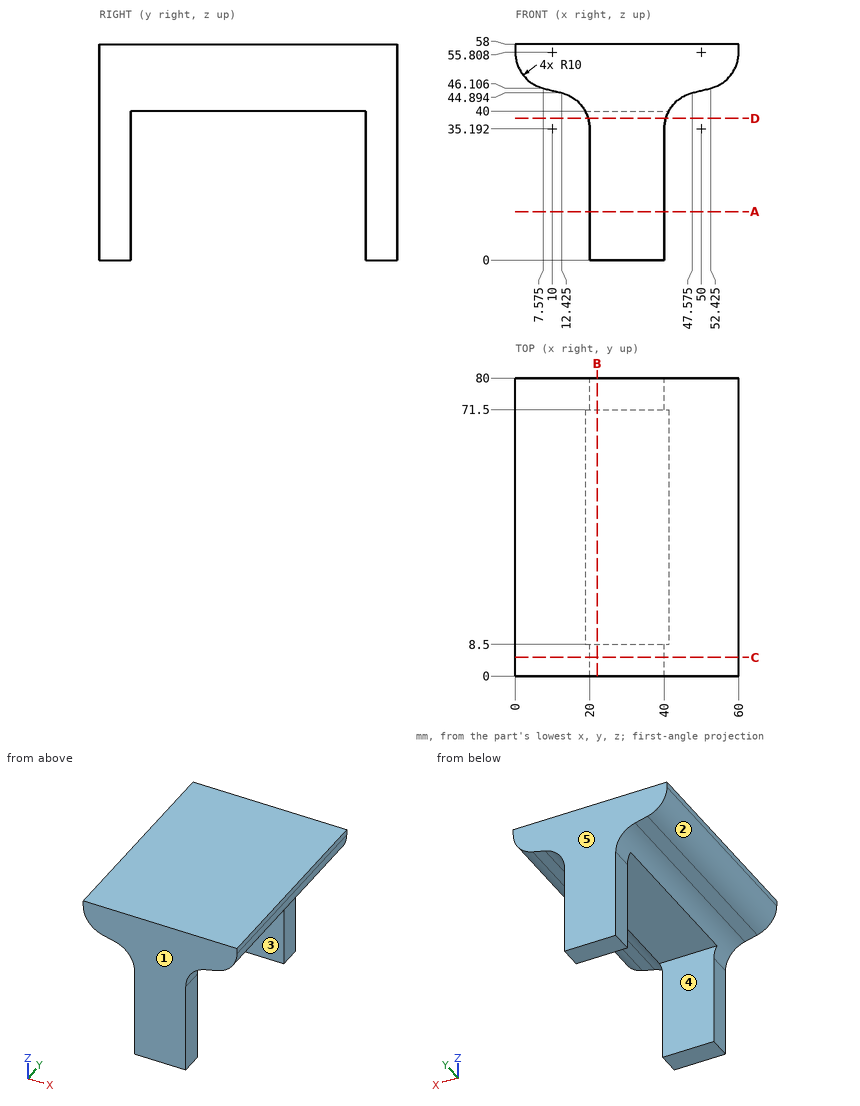
Print and shaded views of the part. All mm, measured from the part's lowest x, y and z. A direction names the side the tool comes from. Give positions to 0.01 mm unless a question says otherwise; leave off trailing zeros. Write each loop counter-clockwise with the first axis right and the second up, starting at its lowest first coordinate (ties: lowest second). Pieces come first, ordered by that corner, then holes. Notation, with made-up numbers: (78.25, 69.25) - (96.25, 69.25) arc R33 cw to (96.25, 99.25) - close; hole circle Ø5 at (79, 32). An arc over 180 degrees is marked (long way). One line per question, with ' | ' between items. Start each with the question number.
(1) Two-plate mould, pull along Y, no slides. Class the marked faces 1, 2 and 3: +Y half, -Y half, draft (parallel to the pull), parting line (faces both ways), or undercut.
(2) Slice it at A-A on z = 13. Write the cut outline in (x, y), plus the area to 3 significant figures.
(3) Slice it at B-B on x = 22. Write the cut outline in (y, z), plus the area to 3 significant figures.
(4) Slice it at D-D on z = 38. Write the cut outline in (x, y).
(5) Slice it at C-C on y = 5. Write the cut outline in (x, z) (1 decimal), plus the area to 3 significant figures.
(6) Wall check: line 1 along Y through (x, z) = (25.5, 23.5); line 2 along Z through (x, y) = (22, 66.5); line 3 along Z through (x, y) = (7.5, 39) (1 decimal). Give the ranges that are in metal, low to high. Write a range as from..to.
(7) Pin check, flat tips, straight feed: P1, Ø18, axis at x = 35, y = 26.5, coming from the -Z side; P2, Ø9.5, axis at y = 75, z = 24.5, coming from the -X side; P3, Ø2.5, axis at y = 77, z = 15, coming from the +X side. Stop position of each tip, or through.
(8) 3-axis set-ups, long thin cutter, end or side, ignore diameter. For the marked faces 4 and 5: which of +Z, -Z, +X, -X, +Y, -Y reach the whole face in a straight line?
Results below:
1) face 1: -Y half | face 2: draft | face 3: undercut
2) outline: (20, 0) - (40, 0) - (40, 8.5) - (20, 8.5) - close; (20, 71.5) - (40, 71.5) - (40, 80) - (20, 80) - close | area: 340 mm^2
3) outline: (0, 0) - (8.5, 0) - (8.5, 40) - (71.5, 40) - (71.5, 0) - (80, 0) - (80, 58) - (0, 58) - close | area: 2,120 mm^2
4) outline: (19.6, 0) - (40.4, 0) - (40.4, 8.5) - (19.6, 8.5) - close; (19.6, 71.5) - (40.4, 71.5) - (40.4, 80) - (19.6, 80) - close
5) outline: (0, 55.8) arc R10 ccw to (7.6, 46.1) - (12.4, 44.9) arc R10 cw to (20, 35.2) - (20, 0) - (40, 0) - (40, 35.2) arc R10 cw to (47.6, 44.9) - (52.4, 46.1) arc R10 ccw to (60, 55.8) - (60, 58) - (0, 58) - close | area: 1,660 mm^2
6) line 1: 0..8.5, 71.5..80 | line 2: 40..58 | line 3: 46.1..58
7) P1: z = 40 | P2: x = 20 | P3: x = 40
8) face 4: -Z, +X, -X | face 5: +Z, -Z, +X, -X, +Y
